Here's the drawing with two shaded views (mm, measured from the low corner). I have some questions. A direction names the side the tool comes from. Round coordinates to 2 decimals unless told otherwise and drop trailing zeros. Order: outer loops, then holes, each group sorted by start corner. A loop starts at its lowest first (then second) coordinate and runs counter-clockwise, first axis right, second up. Notation, with made-up numbers: (9.5, -3.75) -> (33.5, -3.75) arc R11 ccw to (33.5, 8.25) -> close; hole circle Ø7 at (-7.75, 61.5). An arc over 180 degrees is marked (long way). Answer in a Markdown table with one row per item.
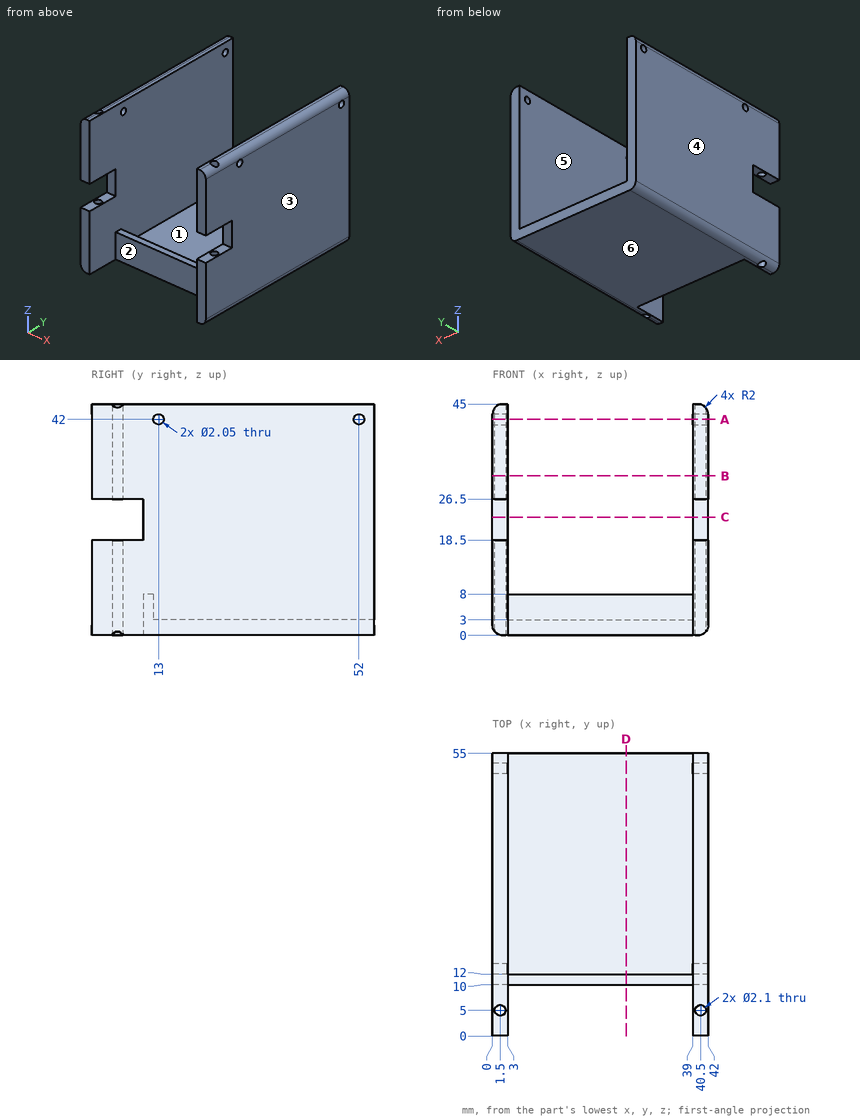
1. Suppose I cut it at B-B on z = 31. Write out the boundary of the cut face in (x, y).
Numbers:
| item | result |
|---|---|
| outline | (0, 0) -> (3, 0) -> (3, 55) -> (0, 55) -> close; (39, 0) -> (42, 0) -> (42, 55) -> (39, 55) -> close; hole circle Ø2.1 at (1.5, 5); hole circle Ø2.1 at (40.5, 5) |
2. We'd pull the mould along X, two halves only. Please class the marked faces 3, 4, 5 and 6: released by +X, released by -X, zero draft, split by the parting line, or undercut.
Numbers:
| item | result |
|---|---|
| face 3 | released by +X |
| face 4 | released by -X |
| face 5 | undercut |
| face 6 | zero draft |
3. For pin 1 Ø1 at (x, y) = (23, 37.5) entering from +Z; pin 2 Ø1.5 at (x, z) = (41, 22) entering from -Y; pin 3 Ø2.5 at (x, z) = (12.5, 5) entering from +Y, each with a flat end and sliding along its axis, tell me the tip position at first contact or that it passes through.
Numbers:
| item | result |
|---|---|
| pin 1 | stops at z = 3 |
| pin 2 | stops at y = 10 |
| pin 3 | stops at y = 12 |
4. Suppose I cut it at A-A on z = 42. Write out the boundary of the cut face in (x, y) (3 decimals), then the cut area to 3 significant figures.
Numbers:
| item | result |
|---|---|
| outline | (0, 0) -> (3, 0) -> (3, 11.975) -> (0, 11.975) -> close; (0, 14.025) -> (3, 14.025) -> (3, 50.975) -> (0, 50.975) -> close; (0, 53.025) -> (3, 53.025) -> (3, 55) -> (0, 55) -> close; (39, 0) -> (42, 0) -> (42, 11.975) -> (39, 11.975) -> close; (39, 14.025) -> (42, 14.025) -> (42, 50.975) -> (39, 50.975) -> close; (39, 53.025) -> (42, 53.025) -> (42, 55) -> (39, 55) -> close; hole circle Ø2.1 at (1.5, 5); hole circle Ø2.1 at (40.5, 5) |
| area | 298 mm2 |
5. Suppose I cut it at D-D on x = 26. Write out the boundary of the cut face in (y, z), then the cut area to 3 significant figures.
Numbers:
| item | result |
|---|---|
| outline | (10, 0) -> (55, 0) -> (55, 3) -> (12, 3) -> (12, 8) -> (10, 8) -> close |
| area | 145 mm2 |
6. Suppose I cut it at C-C on z = 23. Write out the boundary of the cut face in (x, y), then the cut area to 3 significant figures.
Numbers:
| item | result |
|---|---|
| outline | (0, 10) -> (3, 10) -> (3, 55) -> (0, 55) -> close; (39, 10) -> (42, 10) -> (42, 55) -> (39, 55) -> close |
| area | 270 mm2 |
7. For the marked faces 1 and 2, which set-ups out of +Z, -Z, +X, -X, +Y, -Y let a thin tool reach every point of the face, with its end or its side?
Numbers:
| item | result |
|---|---|
| face 1 | +Z, +Y |
| face 2 | +Z, -Z, -Y |
8. Please list where these lines run through material, in increasing order: line 1 along X through (y, z) = (10.5, 32.5); line 2 along Z through (x, y) = (14, 42.5); line 3 along Z through (x, y) = (28.5, 10.5).
Numbers:
| item | result |
|---|---|
| line 1 | x = 0 to 3, 39 to 42 |
| line 2 | z = 0 to 3 |
| line 3 | z = 0 to 8 |
